from build123d import *

# Parameters (mm, degrees)
SKETCH1_R           = 7.5
BOSS_EXTRUDE1_DEPTH = 5


with BuildPart() as part:
    # Sketch1 → Boss-Extrude1 (new, symmetric)
    with BuildSketch(Plane.XY):
        with BuildLine():
            Line((-15, 0), (-15, -30))
            ThreePointArc((-15, -30), (-12.071067812, -37.071067812), (-5, -40))
            Line((-5, -40), (5, -40))
            ThreePointArc((5, -40), (12.071067812, -42.928932188), (15, -50))
            Line((15, -50), (15, -70))
            ThreePointArc((15, -70), (24.609054321, -83.613682099), (40, -90))
            Line((40, -90), (60, -90))
            ThreePointArc((60, -90), (78.236466389, -61.788344037), (45.024841203, -56.743129366))
            ThreePointArc((45.024841203, -56.743129366), (42.350658013, -8.42140399), (0, 15))
            ThreePointArc((0, 15), (-10.606601718, 10.606601718), (-15, 0))
        make_face()
        Circle(SKETCH1_R, mode=Mode.SUBTRACT)
        with Locations((60, -70)):
            Circle(SKETCH1_R, mode=Mode.SUBTRACT)
    extrude(amount=BOSS_EXTRUDE1_DEPTH, both=True)


solid = part.part
Input: part model. Units: mm. Frame: model coordinates. A direction names the side the tool comes from. Give positions to 0.01 mm unless a question says otherwise; leave off trailing zeros. Loops run counter-clockwise (first coordinate to the right, second up) from the corner with the lowest first, then second, coordinate; pieces in that order, holes last. Notation, with made-up numbers: (12.25, 83.25) -> (42.25, 83.25) arc R13 cw to (42.25, 107.25) -> close; hole circle Ø10 at (-8, 20). An arc over 180 degrees is marked (long way). Answer as a JSON object with one key per item and string values. Group by question number.
Item 1: Cut plane C-C, the plane x = 69.5. Return the cut outline in (y, z), and give its area (3 significant figures).
Item 2: Cut plane D-D, the plane y = -25. Return the cut outline in (x, z), and give its area (3 significant figures).
Item 3: Pull-direction query (X, two-part tool) for faces 1 (the cylindrical face through (11.99, -42.85, 0.07)), 2 (the cylindrical face through (52.507, -69.67, -0.07)), 3 (the flat face through (50, -90, 0)); classes: released by +X, released by -X, zero draft, split by the parting line, or undercut.
Item 4: Reachability of faces 4 (the flat face through (32, -37, -5)), 5 (the flat face through (0, -40, 0)) from +Z, -Z, +X, -X, +Y, -Y: full face, straight path, thin tool, end or side. Return the list, or none.
Item 5: Pin query (flat end, axial travel): P1, Ø5, axis at y = -37.5, z = -2.5, coming from the -X side; P2, Ø13.5, axis at x = 0, y = 0, coming from the -Z side; P3, Ø3, axis at y = -18, z = 0, coming from the +X side; P4, Ø1, axis at x = 18.5, z = -1.5, coming from the +Y side. Return the tip coordinate at first contact, or that it passes through.
Item 6: Cut plane A-A, the plane z = 1. Return the cut outline in (x, y), and give its area (3 significant figures).
Item 7: Cut plane B-B, the plane y = -53. Return the cut outline in (x, z), and give its area (3 significant figures).
Item 8: Line query: probe 1 along Y at (x, z) = (60, 2); probe 2 along Y at (x, z) = (0, 1); probe 3 along X at (y, z) = (-53, -0.5). Output: solid intervals per line, ascending.
Checks:
{
 "1": {"outline": "(-87.6, -5) -> (-52.4, -5) -> (-52.4, 5) -> (-87.6, 5) -> close", "area": "352 mm²"},
 "2": {"outline": "(-15, -5) -> (48.99, -5) -> (48.99, 5) -> (-15, 5) -> close", "area": "640 mm²"},
 "3": {"face 1": "released by -X", "face 2": "undercut", "face 3": "zero draft"},
 "4": {"face 4": "-Z, +X, -X, +Y, -Y", "face 5": "+Z, -Z, -X, -Y"},
 "5": {"P1": "stops at x = -13.66", "P2": "passes through", "P3": "stops at x = 47.54", "P4": "stops at y = 11.65"},
 "6": {"outline": "(-15, -30) arc R10 ccw to (-5, -40) -> (5, -40) arc R10 cw to (15, -50) -> (15, -70) arc R30 ccw to (40, -90) -> (60, -90) arc R20 ccw (long way) to (45.02, -56.74) arc R50 ccw to (0, 15) arc R15 ccw to (-15, 0) -> close; hole circle Ø15 at (0, 0); hole circle Ø15 at (60, -70)", "area": "5,230 mm²"},
 "7": {"outline": "(15, -5) -> (46.65, -5) -> (46.65, 5) -> (15, 5) -> close; (49.46, -5) -> (70.54, -5) -> (70.54, 5) -> (49.46, 5) -> close", "area": "527 mm²"},
 "8": {"probe 1": "y = -90 to -77.5, -62.5 to -50", "probe 2": "y = -40 to -7.5, 7.5 to 15", "probe 3": "x = 15 to 46.65, 49.46 to 70.54"}
}
